Part model, mm, in its own coordinate system. Face numbers are marked on the shaded views. A direction names the side the tool comes from. Coordinates: 2 decimals unless noted, no trailing zeros. Order: outer loops, then holes, each group sorted by start corner. A loop starts at its lowest first (then second) coordinate and runs counter-clockwise, first axis right, second up.
1) Pin check, flat tip, straight feed: pin 1 Ø3.5 at (y, z) = (25.5, 0.5) entering from +X. Stop position of the tip, or through.
2) Mould opens along Z. For the marked faces 3, 4 and 5 say: +Z half, -Z half, draft (parallel to the pull), parting line (faces both ways), or undercut.
3) Cut at C-C (z = 3.75). List the corners of the cut face in (x, y).
4) Tool access for the marked faces 1 and 2: list every direction of +Z, -Z, +X, -X, +Y, -Y with a clear straight run to the whole face (end or side of a thin tool).
5) Cut at B-B (y = 8.5). List the corners of the cut face in (x, z), and give its area (3 significant figures).
6) Wall check: L1, parallel to Z at x = -3, y = 13; L2, parallel to Y at x = -0.75, z = -10; L3, parallel to Z at x = 0.5, y = 28.5. Give the ranges that are in metal, low to high.
7) Cut at A-A (x = -0.75). List the corners of the cut face in (y, z).
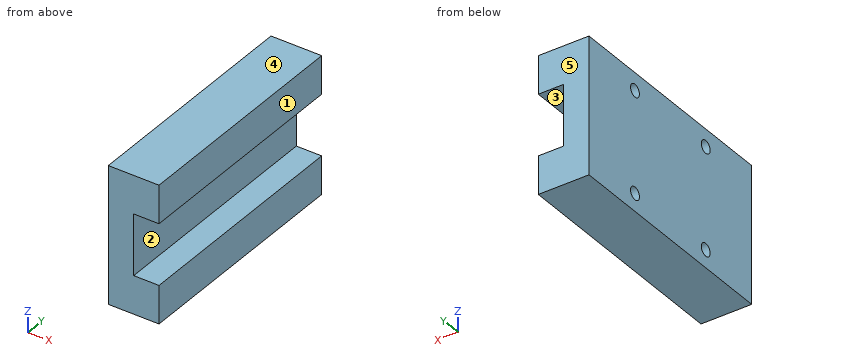
```python
from build123d import *

# Parameters (mm, degrees)
BOSS_EXTRUDE1_DEPTH   = 46
M3_TAPPED_HOLE1_D     = 2.5
M3_TAPPED_HOLE1_DEPTH = 7.5
M3_TAPPED_HOLE1_TIP   = 0.751075774


with BuildPart() as part:
    # Sketch1 → Boss-Extrude1 (new body)
    with BuildSketch(Plane(origin=(0, 0, 0), x_dir=(1, 0, 0), z_dir=(0, 1, 0))):
        Polygon((5, 6), (5, 13.5), (-5, 13.5), (-5, -13.5), (5, -13.5), (5, -6), (0, -6), (0, 6), align=None)
    extrude(amount=BOSS_EXTRUDE1_DEPTH)

    # M3 Tapped Hole1
    with Locations(Plane.ZY.offset(5)):
        with Locations((10, 33), (-10, 33), (-10, 13), (10, 13)):
            Hole(M3_TAPPED_HOLE1_D / 2, depth=M3_TAPPED_HOLE1_DEPTH)
            with Locations((0, 0, -(M3_TAPPED_HOLE1_DEPTH + M3_TAPPED_HOLE1_TIP / 2))):  # 118° drill point
                Cone(0, M3_TAPPED_HOLE1_D / 2, M3_TAPPED_HOLE1_TIP, mode=Mode.SUBTRACT)


solid = part.part
```
Geometry check:
1. pin 1: stops at x = 0
2. face 3: undercut
2. face 4: +Z half
2. face 5: draft
3. outline: (-5, 0) - (0, 0) - (0, 46) - (-5, 46) - close
4. face 1: +Z, -Z, +X, +Y, -Y
4. face 2: +X, +Y, -Y
5. outline: (-5, -13.5) - (5, -13.5) - (5, -6) - (0, -6) - (0, 6) - (5, 6) - (5, 13.5) - (-5, 13.5) - close
5. area: 210 mm2
6. L1: z = -13.5 to -11.25, -8.75 to 8.75, 11.25 to 13.5
6. L2: y = 0 to 11.75, 14.25 to 31.75, 34.25 to 46
6. L3: z = -13.5 to -6, 6 to 13.5
7. outline: (0, -13.5) - (46, -13.5) - (46, 13.5) - (0, 13.5) - close; hole circle Ø2.5 at (13, -10); hole circle Ø2.5 at (13, 10); hole circle Ø2.5 at (33, -10); hole circle Ø2.5 at (33, 10)
